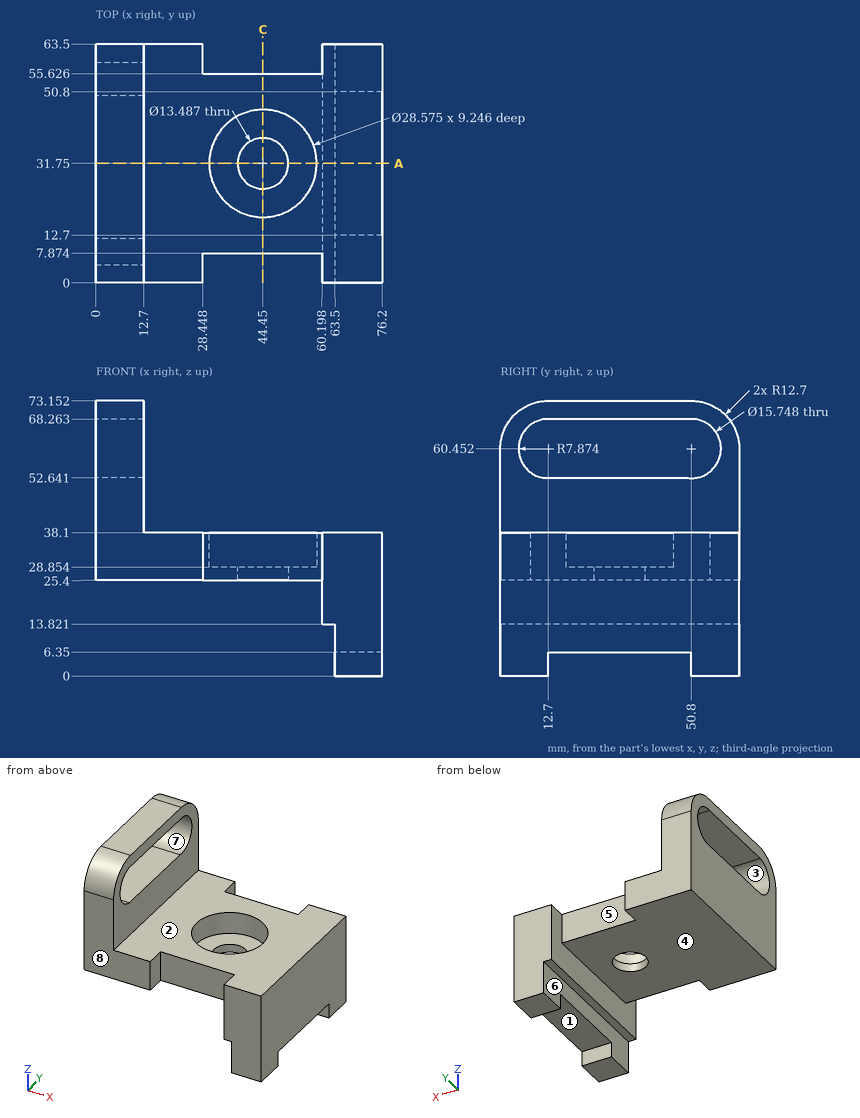
The drawing under review shows one solid part. Ordinate dimensions are in mm from its lowest x, y, z. A direction names the side the tool comes from. Round coordinates to 2 decimals unless told otherwise and drop trailing zeros. Loops run counter-clockwise (first coordinate to the right, second up) from the corner with the lowest first, then second, coordinate; pieces in that order, holes last. Notation, with made-up numbers: (34.25, 67.5) - (67.25, 67.5) arc R15 cw to (67.25, 96.5) - close; hole circle Ø2 at (17.5, 76). An arc over 180 degrees is marked (long way). One line per question, with ' | ' between items.
Q1. Take a section at C-C (x = 44.45). Give the boundary of the cut face in (y, z) (1 decimal), and give its area (3 significant figures).
Taken from the geometry:
outline: (7.9, 25.4) - (25, 25.4) - (25, 28.9) - (17.5, 28.9) - (17.5, 38.1) - (7.9, 38.1) - close; (38.5, 25.4) - (55.6, 25.4) - (55.6, 38.1) - (46, 38.1) - (46, 28.9) - (38.5, 28.9) - close | area: 296 mm²
Q2. The part is to be moulded in two halves that separate along Y. For the marked faces 6, 7 and 8, say which applies: released by +Y, released by -Y, zero draft, split by the parting line, or undercut.
Taken from the geometry:
face 6: zero draft | face 7: undercut | face 8: released by -Y
Q3. For line 1 along Y through (x, z) = (44.45, 35); line 2 along Y through (x, z) = (44.45, 28); line 3 along Z through (x, y) = (8.5, 45), list the stretches that pass through material, from the lowest coordinate up. Write a range as [from, to].
Taken from the geometry:
line 1: y = [7.87, 17.46], [46.04, 55.63] | line 2: y = [7.87, 25.01], [38.49, 55.63] | line 3: z = [25.4, 52.64], [68.26, 73.15]
Q4. Tool access review of the marked faces 1, 2, 3, 4 and 5: name each direction out of +Z, -Z, +X, -X, +Y, -Y from which nothing blocks a thin tool from reaching the whole face with its end or side.
Taken from the geometry:
face 1: -Z, +X, -X | face 2: +Z, +X, +Y, -Y | face 3: +X, -X | face 4: -Z, -X, +Y, -Y | face 5: +Z, -Z, +Y
Q5. Take a section at A-A (y = 31.75). State how many separate pieces and enclosed holes the cut face has, and give its area (3 significant figures).
Taken from the geometry:
separate pieces: 3 | enclosed holes: 0 | area: 1,180 mm²
Q6. For pin 1 (1.5 mm diameter, centred on x = 12, y = 40.5, fed in from -Z); pin 2 (6 mm diameter, centred on x = 30.5, y = 7, fed in from +Z); pin 3 (6 mm diameter, centred on y = 26.5, z = 42, fed in from +X); pin 4 (12.5 mm diameter, centred on y = 50.8, z = 60.452, fed in from +X), all flat-tipped, find the tip position at first contact; note any pin that passes through.
Taken from the geometry:
pin 1: stops at z = 25.4 | pin 2: stops at z = 38.1 | pin 3: stops at x = 12.7 | pin 4: passes through
